Solid Edge part; units mm, degrees
sketch "Sketch1" plane through (0, 0, 0) normal (0, 0, 1) x (1, 0, 0)
  circle A0 centre (0, 0) radius 14
extrude "Protrusion1" add sketch "Sketch1" along normal blind 1
sketch "Sketch2" plane through (0, 0, 1) normal (0, 0, 1) x (1, 0, 0)
  circle A0 centre (0, 0) radius 13
  circle A1 centre (0, 0) radius 14
extrude "Wall" add sketch "Sketch2" along normal blind 4
sketch "Sketch3" plane through (0, 0, 5) normal (0, 0, 1) x (1, 0, 0)
  circle A0 centre (0, 0) radius 15
  circle A1 centre (0, 0) radius 13
extrude "Top" add sketch "Sketch3" along normal blind 2
fillet "Round___Top" radius 2 1 edges at (-15, 0, 7)
sketch "Sketch4" plane through (0, 0, 1) normal (0, 0, 1) x (1, 0, 0)
  line L0 (-9.6593, -2.5882) -> (-7.7274, -2.0706)
  line L1 (-9.6593, 2.5882) -> (-7.7274, 2.0706)
  arc A0 (-9.6593, 2.5882) -> (-9.6593, -2.5882) centre (0, 0) ccw
  arc A1 (-7.7274, -2.0706) -> (-7.7274, 2.0706) centre (0, 0) cw
extrude "Cutout___Alignment" cut sketch "Sketch4" against normal blind 0.5
sketch "Sketch5" plane through (0, 0, 0) normal (0, 0, -1) x (1, 0, 0)
  line L0 (1, -1.5) -> (-1, -1.5)
  line L1 (-1, -1.5) -> (-1, 1.5)
  line L2 (-1, 1.5) -> (1, 1.5)
  line L3 (1, 1.5) -> (1, -1.5)
  dimension "D1" = 1
  dimension "D2" = 1
extrude "Electrics" add sketch "Sketch5" along normal blind 2
sketch "Sketch6" plane through (0, 0, -2) normal (0, 0, -1) x (1, 0, 0)
  line L0 (-1, -1.5) -> (-2, -1.5)
  line L1 (-2, -1.5) -> (-2, 1.5)
  line L2 (-2, 1.5) -> (-1, 1.5)
  line L3 (-1, -1.5) -> (-1, 1.5)
  dimension "D1" = 2
extrude "Wires" add sketch "Sketch6" against normal blind 0.5
hole "Hole1" at (-1.5, -0.7, -2) direction (0, 0, 1) diameter 0.5 end up to next
hole "Hole2" at (-1.5, 0.7, -2) direction (0, 0, 1) diameter 0.5 end up to next
properties material "ABS Plastic, high impact"
Check sheet for the modelled part. Datum: model origin and axes. Units: mm. A direction names the side the tool comes from. Coordinates: 2 decimals unless noted, no trailing zeros. Write each loop counter-clockwise with the first axis right and the second up, starting at its lowest first coordinate (ties: lowest second). Pieces come first, ordered by that corner, then holes.
Item 1: Cross-section at C-C on z = 5.75. Record the boundary of the cut face in (x, y), then the cut area to 3 significant figures.
Numbers:
outline: circle Ø29.71 at (0, 0); hole circle Ø26 at (0, 0)
area: 162 mm2
Item 2: Cross-section at B-B on z = 3.5. Record the boundary of the cut face in (x, y), then the cut area to 3 significant figures.
Numbers:
outline: circle Ø28 at (0, 0); hole circle Ø26 at (0, 0)
area: 84.8 mm2
Item 3: Depth check by flat-ended pin: pin 1 Ø4 at (x, z) = (10, 2) entering from -Y; pin 2 Ø4 at (x, y) = (8, -2.5) entering from -Z; pin 3 Ø0.6 at (x, z) = (-1, -1.5) entering from +Y. Enter the tip coordinate at first touch or a pass-through.
Numbers:
pin 1: stops at y = -11.49
pin 2: stops at z = 0
pin 3: stops at y = 1.5
Item 4: Access from +Z, -Z, +X, -X, +Y, -Y to the whole of each face (thin tool, end or side, straight path). Record for faces 1 (the face through (0, -1.5, -1)), 2 (the face through (-9, 0, 0.5)), 3 (the face through (12.932, 5.362, 2.465)), 4 (the face through (-1, 0, -1)).
Numbers:
face 1: -Z, +X, -X, -Y
face 2: +Z
face 3: -Z
face 4: -X, +Y, -Y
Item 5: Scan lines: probe 1 along Y at (x, z) = (-1.5, -1.85); probe 2 along X at (y, z) = (-0.7, -1.6); probe 3 along Y at (x, z) = (0, 4). Record each from-to range of solid material in increasing order.
Numbers:
probe 1: y = -1.5 to -0.95, -0.45 to 0.45, 0.95 to 1.5
probe 2: x = -2 to -1.75, -1.25 to 1
probe 3: y = -14 to -13, 13 to 14
Item 6: Mould release check, pull along X, two halves, no side actions. Record for faces 5 (the face through (-10.316, 7.91, 3.958)), 6 (the face through (1, 0, -1)), 7 (the face through (0, 1.5, -1)): released by +X, released by -X, zero draft, split by the parting line, or undercut.
Numbers:
face 5: undercut
face 6: released by +X
face 7: zero draft
